Geometry: see drawing. Coordinates: mm, zero at the bounding-box minimum. Coordinates: 2 decimals unless noted, no trailing zeros. Write each loop counter-clockwise with the first axis right and the second up, starting at its lowest first coordinate (ties: lowest second). Pieces come first, ordered by that corner, then holes. Notation, with made-up numbers: M -13.5,55.25 L 4.5,55.25 A20 cw 4.5,63.25 Z; hole C -34,36.5 d4. An arc over 180 degrees is marked long. One line per item, written item: value. Start each with the question number.
Item 1: Mould query, pull axis X, two halves, no side actions, for the marked faces 1, 2 and 3. Classes: released by +X, released by -X, zero draft, split by the parting line, or undercut.
Item 2: Pin query (flat end, axial travel): P1, Ø0.6, axis at y = 4, z = 1, coming from the -X side; P2, Ø0.6, axis at y = 4, z = 0.5, coming from the +X side. Return the tip coordinate at first contact, or that it passes through.
Item 3: Cut plane A-A, the plane z = 9.5. Output: boundary loops of the cut face in (x, y), then the cut area to 3 significant figures.
Item 4: Ray query, L1, parallel to Y at x = 2.9, z = 13.5; L2, parallel to X at y = 2.75, z = 11.5; L3, parallel to Z at x = 4.7, y = 4.4. Return the intervals inside material, ascending. Write a range as from..to.
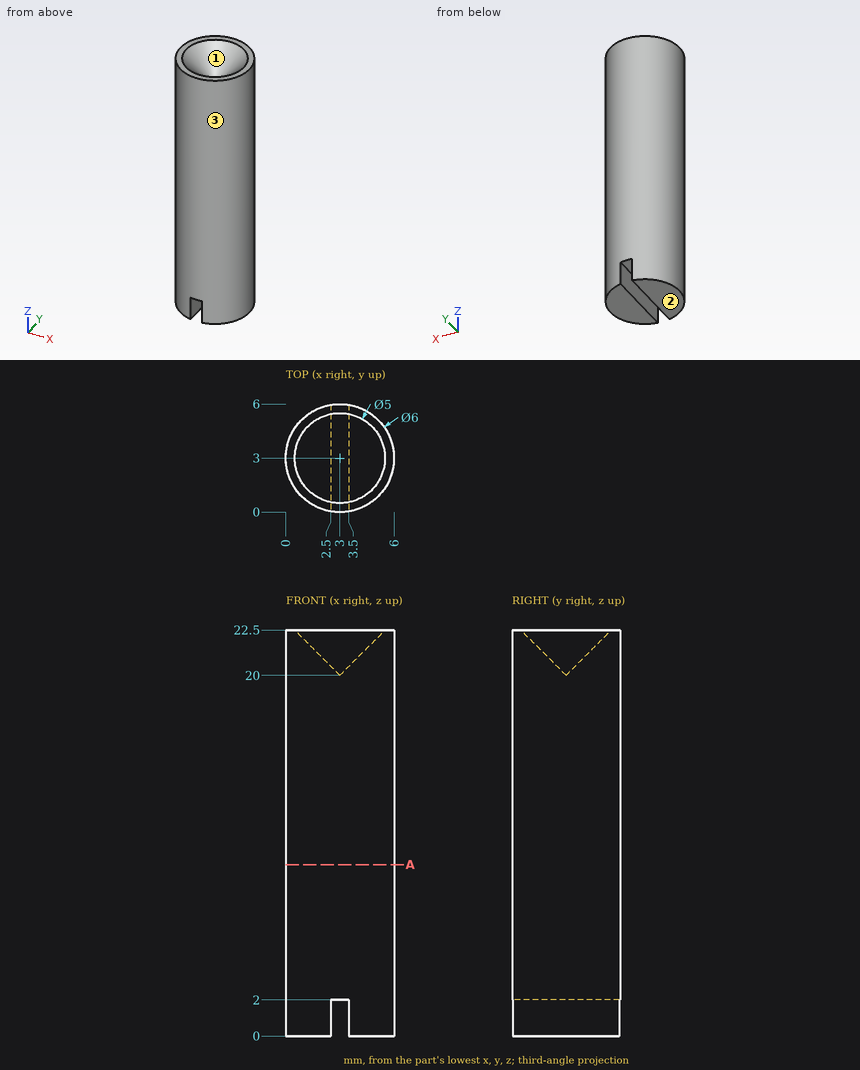
From the geometry:
1. face 1: undercut
1. face 2: zero draft
1. face 3: split by the parting line
2. P1: stops at x = 0.08
2. P2: stops at x = 5.92
3. outline: C 3,3 d6
3. area: 28.3 mm²
4. L1: y = 0..6
4. L2: x = 0.01..5.99
4. L3: z = 0..22.2
